Can you work these out from the drawing? Everything is in mm from the part's minimum corner. A direction names the side the tool comes from. Round coordinates to 2 decimals unless told otherwise and drop trailing zeros. Write each loop counter-clockwise with the first axis right and the second up, starting at its lowest first coordinate (ties: lowest second). Pieces come first, ordered by that corner, then holes. Notation, with made-up numbers: M 41,18 L 82,18 A10 ccw 82,28 Z; hole C 27.5,-35 d10. An arc over 180 degrees is marked long. Answer in a Markdown table with one row per item. Add a question column.
(1) Suppose I cut it at A-A, the plane z = 37.25. Write out the boundary of the cut face in (x, y), then the cut area to 3 significant figures.
(2) Suppose I cut it at D-D, the plane z = 10. Write out the boundary of the cut face in (x, y), then the cut area to 3 significant figures.
(3) I'm going to push flat-ended pins straight in: pin 1 (9.5 mm diameter, centred on x = 9, z = 52, fed in from -Y); pin 2 (3.5 mm diameter, centred on x = 8.5, z = 30, fed in from +Y); pin 3 (3 mm diameter, centred on x = 4.5, z = 27.5, fed in from +Y); pin 4 (3.5 mm diameter, centred on y = 6, z = 32, fed in from +X). Where does each tip first touch, or does it pass through?
(4) Suppose I cut it at B-B, the plane x = 15.25. Write out the boundary of the cut face in (y, z).
(5) If I drill on probe 1 along Z at (x, y) = (8.35, 5.9); probe 2 along Z at (x, y) = (15.35, 39.2); probe 3 along Y at (x, z) = (10, 53), over which ranges is the centre line in solid material (lowest first)?
(6) Suppose I cut it at C-C, the plane x = 8.5. Write out the boundary of the cut face in (y, z).
(7) If we mould it in two halves opening along Z, with no side actions, what happens to the marked faces 5, 6, 7 and 8? For each: released by +Z, released by -Z, zero draft, split by the parting line, or undercut.
(8) For the marked faces 1, 2, 3 and 4, which set-ups out of +Z, -Z, +X, -X, +Y, -Y let a thin tool reach every point of the face, with its end or its side?
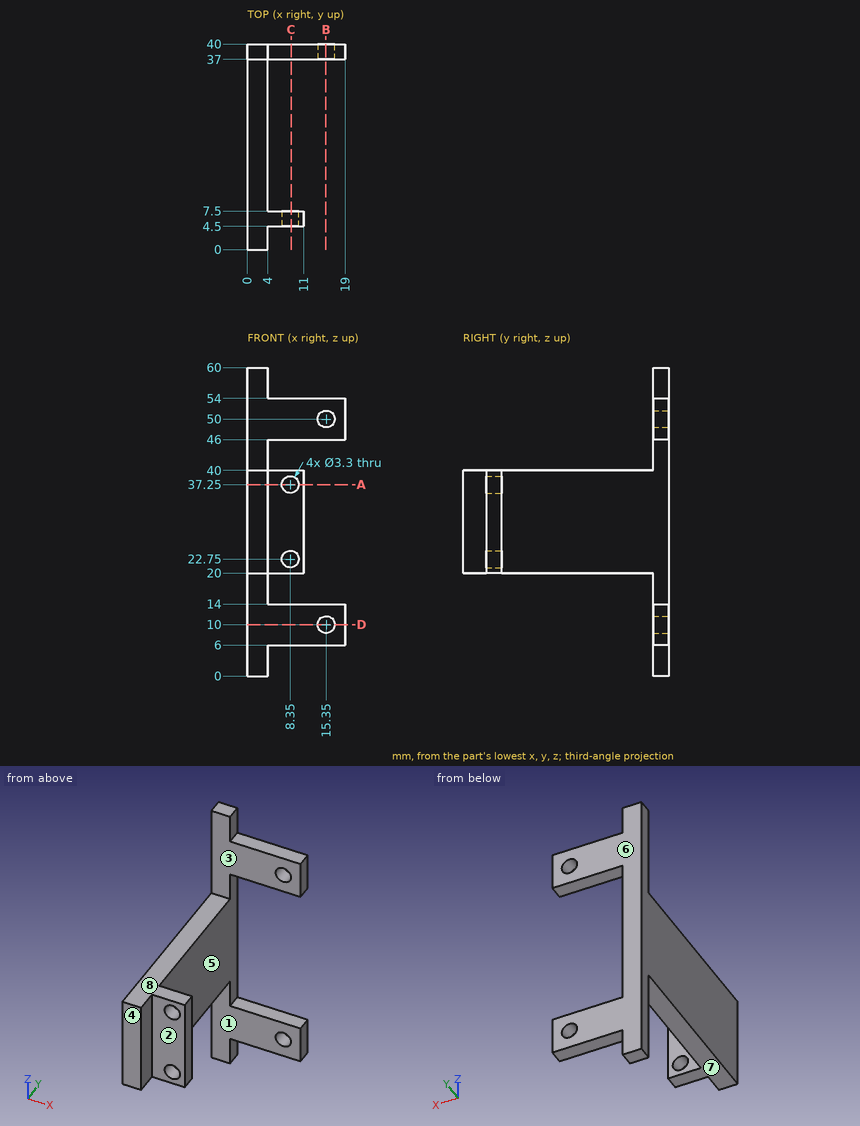
Calculated:
| question | item | result |
|---|---|---|
| 1 | outline | M 0,0 L 4,0 L 4,4.5 L 6.7,4.5 L 6.7,7.5 L 4,7.5 L 4,40 L 0,40 Z; M 10,4.5 L 11,4.5 L 11,7.5 L 10,7.5 Z |
| 1 | area | 171 mm² |
| 2 | outline | M 0,37 L 13.7,37 L 13.7,40 L 0,40 Z; M 17,37 L 19,37 L 19,40 L 17,40 Z |
| 2 | area | 47.1 mm² |
| 3 | pin 1 | y = 37 |
| 3 | pin 2 | y = 7.5 |
| 3 | pin 3 | y = 40 |
| 3 | pin 4 | x = 11 |
| 4 | outline | M 37,6 L 40,6 L 40,8.35 L 37,8.35 Z; M 37,11.65 L 40,11.65 L 40,14 L 37,14 Z; M 37,46 L 40,46 L 40,48.35 L 37,48.35 Z; M 37,51.65 L 40,51.65 L 40,54 L 37,54 Z |
| 5 | probe 1 | 20 to 21.1, 24.4 to 35.6, 38.9 to 40 |
| 5 | probe 2 | 6 to 8.35, 11.65 to 14, 46 to 48.35, 51.65 to 54 |
| 5 | probe 3 | 37 to 40 |
| 6 | outline | M 4.5,20 L 7.5,20 L 7.5,21.11 L 4.5,21.11 Z; M 4.5,24.39 L 7.5,24.39 L 7.5,35.61 L 4.5,35.61 Z; M 4.5,38.89 L 7.5,38.89 L 7.5,40 L 4.5,40 Z; M 37,6 L 40,6 L 40,14 L 37,14 Z; M 37,46 L 40,46 L 40,54 L 37,54 Z |
| 7 | face 5 | undercut |
| 7 | face 6 | zero draft |
| 7 | face 7 | released by -Z |
| 7 | face 8 | released by +Z |
| 8 | face 1 | -Z, +X, -X, -Y |
| 8 | face 2 | +Z, -Z, +X, -Y |
| 8 | face 3 | +Z, +X, -X, -Y |
| 8 | face 4 | +Z, -Z, +X, -X, -Y |
